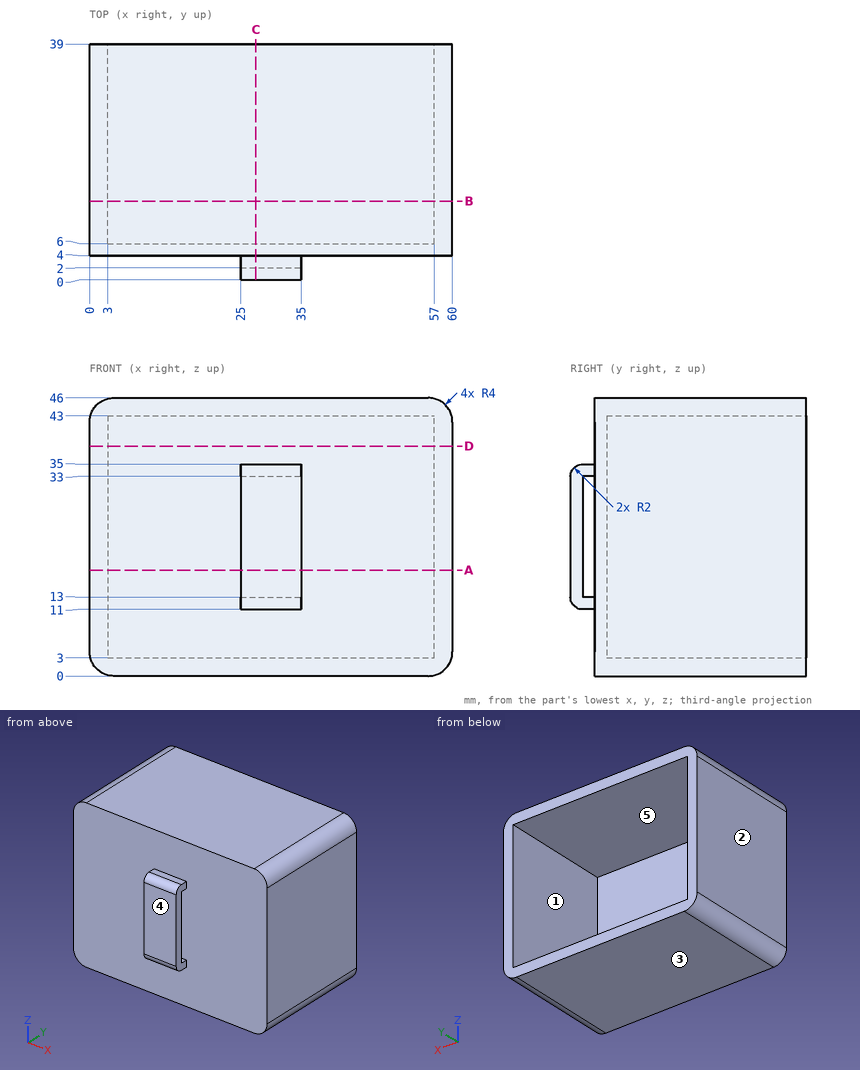
Study the drawing (mm; zero at the part's minimum x, y, z) and answer. A direction names the side the tool comes from. Give positions to 0.01 mm unless a question says otherwise; leave off trailing zeros. Order: outer loops, then holes, each group sorted by start corner. A loop starts at its lowest first (then second) coordinate and runs counter-clockwise, first axis right, second up. Notation, with made-up numbers: M -32,74.5 L 0,74.5 A23 ccw 0,91.5 Z; hole C 67,86 d3. An arc over 180 degrees is marked long. Put each result on its own line as item: value. Start each with the question number.
Item 1: For a pull along Z with two mould halves and no side action, classify the marked faces 3, 4 and 5 as +Z half, -Z half, draft (parallel to the pull), parting line (faces both ways), or undercut.
Item 2: The part is cut by section A-A, the plane z = 17.5. Determine the outline of the cut face in (x, y).
Item 3: The part is cut by section B-B, the plane y = 13. Determine the outline of the cut face in (x, z), and give its area (3 significant figures).
Item 4: Which of the six approach directions +Z, -Z, +X, -X, +Y, -Y give full straight-line access (tool end or side, diameter ignored) to the marked faces 1 and 2?
Item 5: The part is cut by section D-D, the plane z = 38. Determine the outline of the cut face in (x, y).
Item 6: Flat-ended cylindrical pins translate along their axes: P1, Ø1.6, axis at x = 30.5, y = 3, coming from the +Z side; P2, Ø5, axis at x = 30, z = 20.5, coming from the +Y side; P3, Ø6, axis at x = 10, z = 30, coming from the -Y side. Find the tip coordinate at first contact, or state that the pin passes through.
Item 7: The part is cut by section C-C, the plane x = 27.5. Determine the outline of the cut face in (y, z).
Item 8: Find the intervals of material crossed by line 1 along Z through (x, y) = (27.5, 16); line 2 along X through (y, z) = (23, 37.5); line 3 along Y through (x, z) = (15.5, 43.5), in increasing order.
Answer key:
1. face 3: -Z half
1. face 4: draft
1. face 5: undercut
2. outline: M 0,4 L 60,4 L 60,39 L 57,39 L 57,6 L 3,6 L 3,39 L 0,39 Z; M 25,0 L 35,0 L 35,2 L 25,2 Z
3. outline: M 0,4 A4 ccw 4,0 L 56,0 A4 ccw 60,4 L 60,42 A4 ccw 56,46 L 4,46 A4 ccw 0,42 Z; hole M 3,3 L 57,3 L 57,43 L 3,43 Z
3. area: 586 mm²
4. face 1: +Y
4. face 2: +Z, -Z, -X, +Y, -Y
5. outline: M 0,4 L 60,4 L 60,39 L 57,39 L 57,6 L 3,6 L 3,39 L 0,39 Z
6. P1: stops at z = 35
6. P2: stops at y = 6
6. P3: stops at y = 4
7. outline: M 0,13 A2 ccw 2,11 L 4,11 L 4,0 L 39,0 L 39,3 L 6,3 L 6,43 L 39,43 L 39,46 L 4,46 L 4,35 L 2,35 A2 ccw 0,33 Z; hole M 2,13 L 4,13 L 4,33 L 2,33 Z
8. line 1: z = 0 to 3, 43 to 46
8. line 2: x = 0 to 3, 57 to 60
8. line 3: y = 4 to 39
